from build123d import *

# Parameters (mm, degrees)
BOSS_EXTRUDE1_DEPTH     = 15
BOSS_EXTRUDE2_DEPTH     = 70
SKETCH3_W               = 10
SKETCH3_H               = 15
BOSS_EXTRUDE3_DEPTH     = 30
CUT_EXTRUDE1_DEPTH      = 156.563491861
CUT_EXTRUDE1_DEPTH_BACK = 156.563491861
CUT_EXTRUDE2_DEPTH      = 156.563491861
CUT_EXTRUDE2_DEPTH_BACK = 156.563491861
SKETCH5_W               = 40
SKETCH5_H               = 40
BOSS_EXTRUDE4_DEPTH     = 30
CUT_EXTRUDE3_START      = 15
CUT_EXTRUDE3_DEPTH      = 60


with BuildPart() as part:
    # Sketch1 → Boss-Extrude1 (new body)
    with BuildSketch(Plane(origin=(0, 0, 0), x_dir=(1, 0, 0), z_dir=(0, 1, 0))):
        Polygon((0, 0), (0, -20), (40, -70), (120, -70), (120, 0), align=None)
    extrude(amount=BOSS_EXTRUDE1_DEPTH)

    # Sketch2 → Boss-Extrude2 (add)
    with BuildSketch(Plane.XY):
        with BuildLine():
            Line((50, 15), (110, 15))
            Line((110, 15), (110, 28.542486889))
            ThreePointArc((110, 28.542486889), (117.416573868, 40.857864376), (120, 55))
            Line((120, 55), (40, 55))
            ThreePointArc((40, 55), (42.583426132, 40.857864376), (50, 28.542486889))
            Line((50, 28.542486889), (50, 15))
        make_face()
    extrude(amount=BOSS_EXTRUDE2_DEPTH)

    # Sketch3 → Boss-Extrude3 (add)
    with BuildSketch(Plane.XY):
        with Locations((115, 62.5)):
            Rectangle(SKETCH3_W, SKETCH3_H)
    boss_extrude3 = extrude(amount=BOSS_EXTRUDE3_DEPTH)

    # Mirror1: Boss-Extrude3 across plane
    add(boss_extrude3.mirror(Plane(origin=(80, 0, 0), x_dir=(0, 0, 1), z_dir=(1, 0, 0))))

    # Sketch4 → Cut-Extrude1 (cut, two sides: drawn at the far end of the back side and taken through both)
    with BuildSketch(Plane.XY.offset(-CUT_EXTRUDE1_DEPTH_BACK)):
        with BuildLine():
            Line((50, 72), (50, 55))
            ThreePointArc((50, 55), (80, 25), (110, 55))
            Line((110, 55), (110, 72))
            Line((110, 72), (50, 72))
        make_face()
    extrude(amount=CUT_EXTRUDE1_DEPTH + CUT_EXTRUDE1_DEPTH_BACK, mode=Mode.SUBTRACT)

    # Sketch5 → Cut-Extrude2 (cut, two sides: drawn at the far end of the back side and taken through both)
    with BuildSketch(Plane(origin=(0, 0, 0), x_dir=(1, 0, 0), z_dir=(0, 1, 0)).offset(-CUT_EXTRUDE2_DEPTH_BACK)):
        with Locations((80, -30)):
            Rectangle(SKETCH5_W, SKETCH5_H)
    extrude(amount=CUT_EXTRUDE2_DEPTH + CUT_EXTRUDE2_DEPTH_BACK, mode=Mode.SUBTRACT)

    # Sketch6 → Boss-Extrude4 (add)
    with BuildSketch(Plane.XY):
        Polygon((0, 15), (40, 70), (50, 70), (50, 15), align=None)
    extrude(amount=BOSS_EXTRUDE4_DEPTH)

    # Sketch7 → Cut-Extrude3 (cut)
    with BuildSketch(Plane(origin=(0, 0, 0), x_dir=(1, 0, 0), z_dir=(0, 1, 0)).offset(CUT_EXTRUDE3_START)):
        Polygon((0, -20), (40, -30), (0, -30), align=None)
    extrude(amount=CUT_EXTRUDE3_DEPTH, mode=Mode.SUBTRACT)


solid = part.part
Can you work these out from the model? Positions are in its coordinate system, mm. A direction names the side the tool comes from. Coordinates: 2 decimals unless noted, no trailing zeros. Loops run counter-clockwise (first coordinate to the right, second up) from the corner with the lowest first, then second, coordinate; pieces in that order, holes last. Notation, with made-up numbers: M 75,29 L 85,29 A14 cw 85,53 Z; hole C -23,89 d2. An arc over 180 degrees is marked long. Return JSON: item names as keys, results as strings. Group by question number.
Item 1: Imagine slicing it at B-B (x = 80). Please give me the cut outline in (y, z).
Item 2: Imagine slicing it at A-A (z = 40). Please give me the cut outline in (x, y).
Item 3: On a 3-axis mill with a long thin cutter (end or side, diameter ignored), from which of +Z, -Z, +X, -X, +Y, -Y can I reach the whole of each face in a straight line? I mean faces 4 (the flat face through (120, 62, 15)), 5 (the flat face through (50, 62, 15)), 6 (the flat face through (115, 55, 50)), 7 (the flat face through (100, 16, 30)), 8 (the cylindrical face through (42.51, 41.05, 49.72)). Say none if no direction works.
Item 4: If I drill on L1, parallel to Z at x = 88, y = 11; L2, parallel to Z at x = 40, y = 55; L3, parallel to X at y = 46, z = 45, over which ranges is the centre line in solid material (lowest first)? Write a range as from..to.
Item 5: Imagine slicing it at D-D (z = 62.5). Please give me the cut outline in (x, y), and give its area (3 significant figures).
Item 6: I'm going to push flat-ended pins straight in: pin 1 Ø1.5 at (x, z) = (102.5, 34.5) entering from -Y; pin 2 Ø15 at (y, z) = (24.5, 49.5) entering from -X; pin 3 Ø3 at (x, z) = (47, 55.5) entering from +Y; pin 4 Ø3 at (x, y) = (45.5, 29.5) entering from +Z. Where does each tip first touch, or does it pass through?
Item 7: Imagine slicing it at C-C (y = 64). Please give me the cut outline in (x, z).
Item 8: Thinking about a two-plate mould opening in X: for faces 1 (the flat face through (110, 22, 35)), 2 (the flat face through (44, 26, 30)), 3 (the flat face through (80, 12, 50)), which applies, released by +X, released by -X, zero draft, split by the parting line, or undercut?
Verdict:
{
 "1": {"outline": "M 0,0 L 25,0 L 25,10 L 0,10 Z; M 0,50 L 25,50 L 25,70 L 0,70 Z"},
 "2": {"outline": "M 16,0 L 60,0 L 60,32.64 A30 cw 50,55 L 40,55 A40 ccw 50,28.54 L 50,15 L 16,15 Z; M 100,0 L 120,0 L 120,15 L 110,15 L 110,28.54 A40 ccw 120,55 L 110,55 A30 cw 100,32.64 Z"},
 "3": {"face 4": "+Z, -Z, +X, +Y, -Y", "face 5": "+Z, -Z, +Y", "face 6": "+Z, +X, -X, +Y", "face 7": "+Y, -Y", "face 8": "+Z, -X"},
 "4": {"L1": "z = 0..10, 50..70", "L2": "z = 0..30", "L3": "x = 41.03..51.38, 108.62..118.97"},
 "5": {"outline": "M 34,0 L 120,0 L 120,15 L 110,15 L 110,28.54 A40 ccw 120,55 L 110,55 A30 cw 50,55 L 40,55 A40 ccw 50,28.54 L 50,15 L 34,15 Z", "area": "2,640 mm^2"},
 "6": {"pin 1": "stops at y = 0", "pin 2": "stops at x = 47.27", "pin 3": "stops at y = 55", "pin 4": "stops at z = 30"},
 "7": {"outline": "M 35.64,0 L 50,0 L 50,30 L 40,30 L 35.64,28.91 Z; M 110,0 L 120,0 L 120,30 L 110,30 Z"},
 "8": {"face 1": "released by +X", "face 2": "zero draft", "face 3": "undercut"}
}
